Autodesk Inventor part; units mm, degrees
ref_plane "YZ Plane" through (0, 0, 0) normal (1, 0, 0) x (0, 1, 0)
ref_plane "XZ Plane" through (0, 0, 0) normal (0, 1, 0) x (-1, 0, 0)
ref_plane "XY Plane" through (0, 0, 0) normal (0, 0, 1) x (1, 0, 0)
sketch "Sketch1" plane through (0, 0, 0) normal (0, 0, 1) x (1, 0, 0)
  line L0 (-51.3998, 21.3475) -> (-0.5998, 21.3475)
  line L1 (-0.5998, 21.3475) -> (-0.5998, -80.2525)
  line L2 (-0.5998, -80.2525) -> (-25.9998, -80.2525)
  line L3 (-25.9998, -80.2525) -> (-51.3998, -4.0525)
  line L4 (-51.3998, -4.0525) -> (-51.3998, 21.3475)
  dimension "d1" = 50.8
  dimension "d3" = 25.4
  dimension "d4" = 76.2
  dimension "d5" = 25.4
extrude "Extrusion1" add sketch "Sketch1" along normal blind 19.05
sketch "Sketch2" plane through (-51.3998, 21.3475, 0) normal (0, 1, 0) x (1, 0, 0)
  line L0 (0, 0) -> (50.8, 0)
  line L1 (38.1, 0) -> (44.45, 0)
  line L2 (44.45, 0) -> (44.45, -12.7)
  line L3 (44.45, -12.7) -> (38.1, -12.7)
  line L4 (38.1, -12.7) -> (38.1, 0)
  line L5 (50.8, 0) -> (50.8, -19.05)
  point P0 (51.3998, 0)
  dimension "d8" = 6.35
  dimension "d10" = 6.35
  dimension "d11" = 12.7
extrude "Extrusion2" cut sketch "Sketch2" against normal blind 101.6
fillet "Fillet1" radius 3.175 3 edges at (-0.5998, -29.4525, 19.05) (-38.6998, -42.1525, 19.05) (-51.3998, 8.6475, 19.05)
equation "\"d12\" = d5 + d4"
properties part number "Right Leg, Front part"
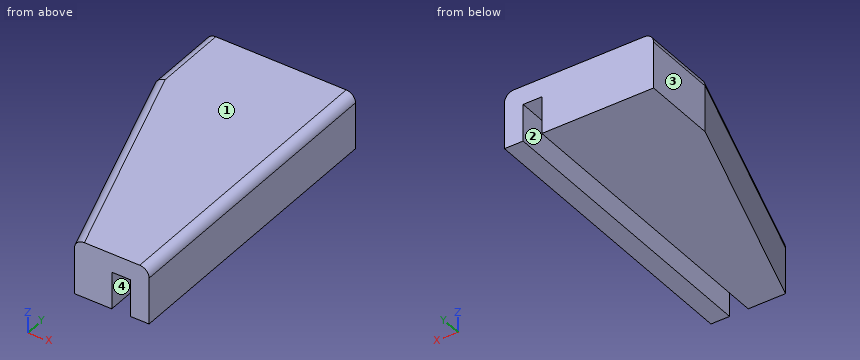
Model file for the job. Use its own axes, mm. Face numbers are marked on the shaded views. Give positions to 0.01 mm unless a question says otherwise; leave off trailing zeros. Write each loop counter-clockwise with the first axis right and the second up, starting at its lowest first coordinate (ties: lowest second). Pieces come first, ordered by that corner, then holes. Notation, with made-up numbers: (61, -38) - (70, -38) arc R22 ccw to (70, -29) - close; hole circle Ø10 at (76, 82.25). An arc over 180 degrees is marked (long way). Answer as CSV lines item,"result".
1. Two-plate mould, pull along X, no slides. Class the marked faces 1, 2, 3 and 4: +X half, -X half, draft (parallel to the pull), parting line (faces both ways), or undercut.
Responses:
face 1,"draft"
face 2,"undercut"
face 3,"-X half"
face 4,"undercut"
2. Band-saw the part on C-C (x = -10). Write the cut outline in (y, z).
Responses:
outline,"(-80.25, 12.7) - (21.35, 12.7) - (21.35, 19.05) - (-80.25, 19.05) - close"
3. Band-saw the part on A-A (z = 8.25). Write the cut outline in (x, y).
Responses:
outline,"(-51.4, -4.05) - (-26, -80.25) - (-13.3, -80.25) - (-13.3, 21.35) - (-51.4, 21.35) - close; (-6.95, -80.25) - (-0.6, -80.25) - (-0.6, 21.35) - (-6.95, 21.35) - close"
4. Band-saw the part on B-B (z = 14.5). Write the cut outline in (x, y).
Responses:
outline,"(-51.4, -4.05) - (-26, -80.25) - (-0.6, -80.25) - (-0.6, 21.35) - (-51.4, 21.35) - close"
5. Drill centre lines: L1, parallel to X at y = -1.5, z = 6; L2, parallel to X at y = -14.5, z = 1.5; L3, parallel to X at y = 1.5, z = 16.25. Where is each one in solid material? Low to high. Write a range as [from, to].
Responses:
L1,"x = [-51.4, -13.3], [-6.95, -0.6]"
L2,"x = [-47.92, -13.3], [-6.95, -0.6]"
L3,"x = [-51.38, -0.62]"
6. Pin check, flat tip, straight feed: pin 1 (4 mm diameter, centred on y = -19.5, z = 9, fed in from -X). Stop position of the tip, or through.
Responses:
pin 1,"stops at x = -46.92"
